```python
from build123d import *

# Parameters (mm, degrees)
F0_W     = 70.443585515
F0_H     = 70.443585515
F1_DEPTH = 30


# Not quite as in the source:
# - a feature names something its author has since deleted; it is built from what else it names


with BuildPart() as f1:
    # F0 (on Top) → F1 (new body)
    with BuildSketch(Plane.XY):
        Rectangle(F0_W, F0_H)
    extrude(amount=-F1_DEPTH)

    # F2 (on Front) → F3 (revolve, cut)
    with BuildSketch(Plane.XZ):
        with BuildLine():
            Line((0, -7), (0, -16))
            Line((0, -16), (0, -25.8))
            ThreePointArc((0, -25.8), (14.8091399143, -23.279001082), (27.95, -16))
            Line((27.95, -16), (28.45, -7))
            Line((28.45, -7), (28.6166666667, -4))
            Line((28.6166666667, -4), (28.6166666667, 0))
            Line((28.6166666667, 0), (0, 0))
            Line((0, 0), (0, -4))
            Line((0, -4), (0, -7))
        make_face()
    revolve(axis=Axis((0, 0, -11.5), (0, 0, 1)), mode=Mode.SUBTRACT)


solid = f1.part
```
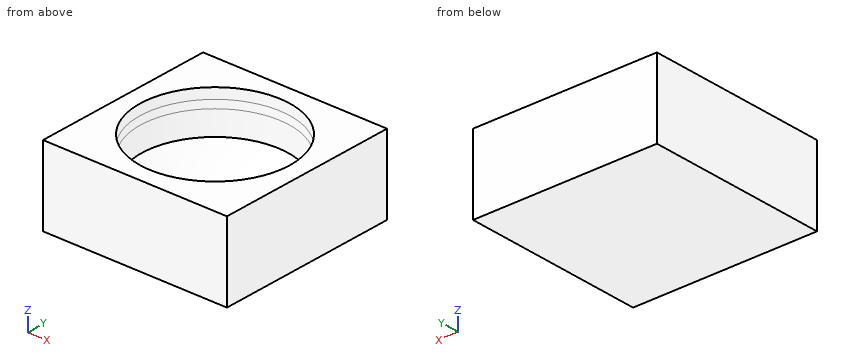
Here's how the part is built. I have some questions about the finished solid (model axes, mm). Coordinates: 2 decimals unless noted, no trailing zeros. Loops run counter-clockwise (first coordinate to the right, second up) from the corner with the lowest first, then second, coordinate; pieces in that order, holes last. Notation, with made-up numbers: M 44,8 L 98,8 A27 cw 98,35 Z; hole C 4.25,56 d7. An arc over 180 degrees is marked long. One line per item, written item: value.
1. Imagine slicing it at B-B (z = -13.75). List the corners of the cut face in (x, y) for me (3 decimals).
Geometry says:
outline: M -35.222,-35.222 L 35.222,-35.222 L 35.222,35.222 L -35.222,35.222 Z; hole C 0,0 d56.15
2. Imagine slicing it at A-A (z = -21.5). List the corners of the cut face in (x, y) for me, and give its area (3 significant figures).
Geometry says:
outline: M -35.22,-35.22 L 35.22,-35.22 L 35.22,35.22 L -35.22,35.22 Z; hole C 0,0 d38.28
area: 3,810 mm2
3. Please list where these lines run through material, in increasing order: probe 1 along Y at (x, z) = (0, -1.9); probe 2 along X at (y, z) = (22, -9.5); probe 3 along Y at (x, z) = (14, -15.5).
Geometry says:
probe 1: y = -35.22 to -28.62, 28.62 to 35.22
probe 2: x = -35.22 to -17.82, 17.82 to 35.22
probe 3: y = -35.22 to -24.22, 24.22 to 35.22
